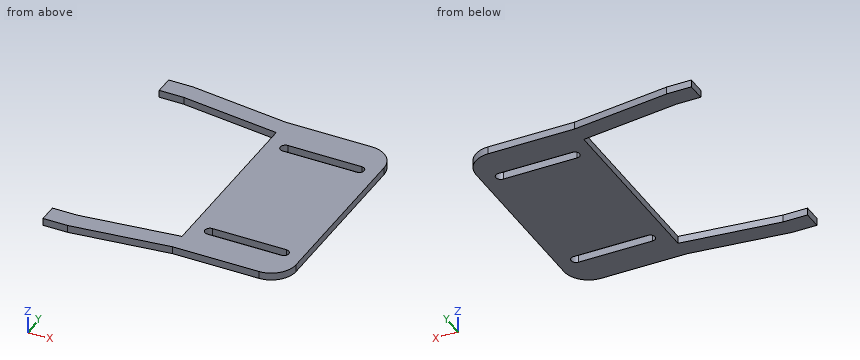
from build123d import *

# Parameters (mm, degrees)
F1_DEPTH = 3


with BuildPart() as f1:
    # F0 (on Top) → F1 (new body)
    with BuildSketch(Plane.XY):
        with BuildLine():
            ThreePointArc((54.314782, 36.214286), (51.38585, 43.285354), (44.314782, 46.214286))
            Line((44.314782, 46.214286), (9.314782, 46.214286))
            Line((9.314782, 46.214286), (-30.685218, 51.214286))
            Line((-30.685218, 51.214286), (-40.685218, 51.214286))
            Line((-40.685218, 51.214286), (-40.685218, 43.714286))
            Line((-40.685218, 43.714286), (-30.685218, 43.714286))
            Line((-30.685218, 43.714286), (9.314782, 38.714286))
            Line((9.314782, 38.714286), (9.314782, -36.285714))
            Line((9.314782, -36.285714), (-30.685218, -41.285714))
            Line((-30.685218, -41.285714), (-40.685218, -41.285714))
            Line((-40.685218, -41.285714), (-40.685218, -48.785714))
            Line((-40.685218, -48.785714), (-30.685218, -48.785714))
            Line((-30.685218, -48.785714), (9.314782, -43.785714))
            Line((9.314782, -43.785714), (44.314782, -43.785714))
            ThreePointArc((44.314782, -43.785714), (51.38585, -40.856782), (54.314782, -33.785714))
            Line((54.314782, -33.785714), (54.314782, 36.214286))
        make_face()
        with BuildLine():
            Line((46.814782, -30.785714), (16.814782, -30.785714))
            ThreePointArc((16.814782, -30.785714), (14.814782, -28.785714), (16.814782, -26.785714))
            Line((16.814782, -26.785714), (46.814782, -26.785714))
            ThreePointArc((46.814782, -26.785714), (48.814782, -28.785714), (46.814782, -30.785714))
        make_face(mode=Mode.SUBTRACT)
        with BuildLine():
            ThreePointArc((46.814782, 33.214286), (48.814782, 31.214286), (46.814782, 29.214286))
            Line((46.814782, 29.214286), (16.814782, 29.214286))
            ThreePointArc((16.814782, 29.214286), (14.814782, 31.214286), (16.814782, 33.214286))
            Line((16.814782, 33.214286), (46.814782, 33.214286))
        make_face(mode=Mode.SUBTRACT)
    extrude(amount=F1_DEPTH)


solid = f1.part
Build history of the part. All positions in model axes, mm. Round coordinates to 2 decimals unless told otherwise and drop trailing zeros. Loops run counter-clockwise (first coordinate to the right, second up) from the corner with the lowest first, then second, coordinate; pieces in that order, holes last. Notation, with made-up numbers: (37, -24.75) -> (63, -24.75) arc R24 ccw to (63, 13.25) -> close; hole circle Ø5 at (21, 40). An arc over 180 degrees is marked (long way). Answer in a Markdown table with one row per item.
Item 1: Saw through at A-A (x = 33). Write the cut outline in (y, z).
Answers below:
| item | result |
|---|---|
| outline | (-43.79, 0) -> (-30.79, 0) -> (-30.79, 3) -> (-43.79, 3) -> close; (-26.79, 0) -> (29.21, 0) -> (29.21, 3) -> (-26.79, 3) -> close; (33.21, 0) -> (46.21, 0) -> (46.21, 3) -> (33.21, 3) -> close |
Item 2: Saw through at B-B (z = 1.85). Write the cut outline in (x, y).
Answers below:
| item | result |
|---|---|
| outline | (-40.69, -48.79) -> (-30.69, -48.79) -> (9.31, -43.79) -> (44.31, -43.79) arc R10 ccw to (54.31, -33.79) -> (54.31, 36.21) arc R10 ccw to (44.31, 46.21) -> (9.31, 46.21) -> (-30.69, 51.21) -> (-40.69, 51.21) -> (-40.69, 43.71) -> (-30.69, 43.71) -> (9.31, 38.71) -> (9.31, -36.29) -> (-30.69, -41.29) -> (-40.69, -41.29) -> close; hole (16.81, -30.79) -> (46.81, -30.79) arc R2 ccw to (46.81, -26.79) -> (16.81, -26.79) arc R2 ccw to start; hole (16.81, 29.21) -> (46.81, 29.21) arc R2 ccw to (46.81, 33.21) -> (16.81, 33.21) arc R2 ccw to start |
Item 3: Pin check, flat tips, straight feed: pin 1 (0.9 mm diameter, centred on x = 25, z = 2, fed in from -Y); pin 2 (1.5 mm diameter, centred on x = 29, z = 2, fed in from +Y); pin 3 (1 mm diameter, centred on y = 16.5, z = 0.5, fed in from -X). Stop position of each tip, or through.
Answers below:
| item | result |
|---|---|
| pin 1 | stops at y = -43.79 |
| pin 2 | stops at y = 46.21 |
| pin 3 | stops at x = 9.31 |
Item 4: Saw through at D-D (y = -32). Write the cut outline in (x, z).
Answers below:
| item | result |
|---|---|
| outline | (9.31, 0) -> (54.31, 0) -> (54.31, 3) -> (9.31, 3) -> close |
Item 5: Saw through at C-C (x = 6). Write the cut outline in (y, z), and give its area (3 significant figures).
Answers below:
| item | result |
|---|---|
| outline | (-44.2, 0) -> (-36.7, 0) -> (-36.7, 3) -> (-44.2, 3) -> close; (39.13, 0) -> (46.63, 0) -> (46.63, 3) -> (39.13, 3) -> close |
| area | 45.0 mm² |
Item 6: Drill centre lines: L1, parallel to Y at x = 24, z = 1.4; L2, parallel to Y at x = -33.5, z = 1.95; L3, parallel to X at y = -1.5, z = 0.5. Where is each one in solid material? Low to high. Write a range as [from, to].
Answers below:
| item | result |
|---|---|
| L1 | y = [-43.79, -30.79], [-26.79, 29.21], [33.21, 46.21] |
| L2 | y = [-48.79, -41.29], [43.71, 51.21] |
| L3 | x = [9.31, 54.31] |
